from build123d import *

# Parameters (mm, degrees)
F0_W          = 101.6
F0_H          = 25.4
F0_R          = 3.3782
F1_DEPTH      = 38.1
F2_R          = 14.2875
F3_DEPTH      = 25.4
F4_W          = 19.05
F4_H          = 31.75
F5_DEPTH      = 50.801
F5_DEPTH_BACK = 50.801


# Not quite as in the source:
# - a feature names something its author has since deleted; it is built from what else it names


with BuildPart() as f1:
    # F0 (on Top) → F1 (new body)
    with BuildSketch(Plane.XY):
        Rectangle(F0_W, F0_H)
        with Locations((-38.1, 0)):
            Circle(F0_R, mode=Mode.SUBTRACT)
        with Locations((38.1, 0)):
            Circle(F0_R, mode=Mode.SUBTRACT)
    extrude(amount=F1_DEPTH)

    # F2 (on face) → F3 (cut)
    with BuildSketch(Plane.XZ.offset(12.7)):
        with Locations((0, 20.6375)):
            Circle(F2_R)
    extrude(amount=-F3_DEPTH, mode=Mode.SUBTRACT)

    # F4 (on Right) → F5 (cut, two sides)
    with BuildSketch(Plane.YZ) as f5_sk:
        with Locations((0, 19.05)):
            Rectangle(F4_W, F4_H)
    extrude(amount=-F5_DEPTH, mode=Mode.SUBTRACT)
    extrude(f5_sk.sketch, amount=F5_DEPTH_BACK, mode=Mode.SUBTRACT)


solid = f1.part
Work out the finished part from the listing and answer in its coordinate system (mm). A direction names the side the tool comes from. Give positions to 0.01 mm unless a question says otherwise; leave off trailing zeros. Write each loop counter-clockwise with the first axis right and the second up, starting at its lowest first coordinate (ties: lowest second). Pieces come first, ordered by that corner, then holes.
Q1. The part is cut by section C-C on z = 13.5. Give the vertices of the cut face in (x, y) (3 decimals).
Answer:
outline: (-50.8, -12.7) - (-12.377, -12.7) - (-12.377, -9.525) - (-50.8, -9.525) - close; (-50.8, 9.525) - (-12.377, 9.525) - (-12.377, 12.7) - (-50.8, 12.7) - close; (12.377, -12.7) - (50.8, -12.7) - (50.8, -9.525) - (12.377, -9.525) - close; (12.377, 9.525) - (50.8, 9.525) - (50.8, 12.7) - (12.377, 12.7) - close
Q2. The part is cut by section A-A on x = -38.1. Give the vertices of the cut face in (y, z) (3 decimals), and give its area (3 significant figures).
Answer:
outline: (-12.7, 0) - (-3.378, 0) - (-3.378, 3.175) - (-9.525, 3.175) - (-9.525, 34.925) - (-3.378, 34.925) - (-3.378, 38.1) - (-12.7, 38.1) - close; (3.378, 0) - (12.7, 0) - (12.7, 38.1) - (3.378, 38.1) - (3.378, 34.925) - (9.525, 34.925) - (9.525, 3.175) - (3.378, 3.175) - close
area: 320 mm2
Q3. A tool of negligible diameter and unlimited length cuts with its end or side. For faces 1 (the face through (-1, -12.7, 6)), 2 (the face through (12, 9.525, 12)), from which of +Z, -Z, +X, -X, +Y, -Y can it reach the whole face along a straight path? Write none if from no direction.
Answer:
face 1: +Z, -Z, +X, -X, -Y
face 2: +X, -X
Q4. The part is cut by section B-B on y = 4.5. Give the vertices of the cut face in (x, z) (3 decimals), and give its area (3 significant figures).
Answer:
outline: (-50.8, 0) - (50.8, 0) - (50.8, 3.175) - (-50.8, 3.175) - close; (-50.8, 34.925) - (50.8, 34.925) - (50.8, 38.1) - (-50.8, 38.1) - close
area: 645 mm2
Q5. For a pull along Z with two mould halves and no side action, classify faces 3 (the face through (-1, 12.7, 6)), 4 (the face through (-1, 0, 0)), 5 (the face through (1, 0, 34.925)), 6 (the face through (-1, 0, 38.1)) as released by +Z, released by -Z, zero draft, split by the parting line, or undercut.
Answer:
face 3: zero draft
face 4: released by -Z
face 5: undercut
face 6: released by +Z
Q6. Straight lines are drawn through the part: L1, parallel to Z at x = -39, y = -7 (3 decimals); L2, parallel to Y at x = -21, z = 5.5 (3 decimals); L3, parallel to Y at x = 38.1, z = 1.8. For each, find the intervals that lie inside material, in ascending order.
Answer:
L1: z = 0 to 3.175, 34.925 to 38.1
L2: y = -12.7 to -9.525, 9.525 to 12.7
L3: y = -12.7 to -3.38, 3.38 to 12.7
Q7. The part is cut by section D-D on y = -2. Give the vertices of the cut face in (x, z) (3 decimals), and give its area (3 significant figures).
Answer:
outline: (-50.8, 0) - (-40.823, 0) - (-40.823, 3.175) - (-50.8, 3.175) - close; (-50.8, 34.925) - (-40.823, 34.925) - (-40.823, 38.1) - (-50.8, 38.1) - close; (-35.377, 0) - (35.377, 0) - (35.377, 3.175) - (-35.377, 3.175) - close; (-35.377, 34.925) - (35.377, 34.925) - (35.377, 38.1) - (-35.377, 38.1) - close; (40.823, 0) - (50.8, 0) - (50.8, 3.175) - (40.823, 3.175) - close; (40.823, 34.925) - (50.8, 34.925) - (50.8, 38.1) - (40.823, 38.1) - close
area: 576 mm2
